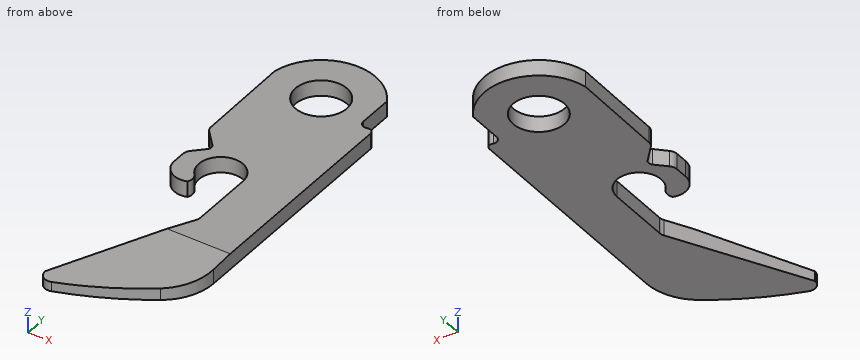
```python
from build123d import *

# Parameters (mm, degrees)
BOSS_EXTRUDE1_DEPTH = 1.27
SKETCH2_R           = 2.0701
CUT_EXTRUDE1_DEPTH  = 2.27
FILLET1_R           = 0.762
CUT_EXTRUDE2_DEPTH  = 10.452014607


with BuildPart() as part:
    # Sketch1 → Boss-Extrude1 (new body)
    with BuildSketch(Plane.XY):
        with BuildLine():
            Line((70.232354199, 59.177106463), (70.232354199, 40.597101988))
            ThreePointArc((70.232354199, 40.597101988), (69.734336591, 38.583930727), (68.355161738, 37.035138686))
            ThreePointArc((68.355161738, 37.035138686), (65.183135809, 35.174825007), (61.781607592, 33.777641675))
            ThreePointArc((61.781607592, 33.777641675), (61.096065134, 33.883458799), (60.780339592, 34.501101988))
            Line((60.780339592, 34.501101988), (66.266739592, 44.661101988))
            Line((66.266739592, 44.661101988), (66.266739592, 44.697700386))
            Line((66.266739592, 44.697700386), (66.266739592, 49.893501988))
            ThreePointArc((66.266739592, 49.893501988), (63.861714839, 51.557269988), (63.152989358, 48.720021988))
            ThreePointArc((63.152989358, 48.720021988), (63.340826318, 48.267953364), (63.214864671, 47.794896889))
            ThreePointArc((63.214864671, 47.794896889), (61.829181489, 47.989948212), (61.186739592, 49.233101988))
            Line((61.186739592, 49.233101988), (61.186739592, 50.249101988))
            ThreePointArc((61.186739592, 50.249101988), (61.245267671, 50.541969288), (61.411860998, 50.789847191))
            Line((61.411860998, 50.789847191), (62.237339742, 51.609423334))
            ThreePointArc((62.237339742, 51.609423334), (62.358185527, 51.888348141), (62.253539592, 52.173746074))
            Line((62.253539592, 52.173746074), (61.016973645, 53.551101988))
            Line((61.016973645, 53.551101988), (60.932739592, 61.477883946))
            ThreePointArc((60.932739592, 61.477883946), (64.518060362, 64.995788774), (69.060739592, 62.852369819))
            Line((69.060739592, 62.852369819), (69.060739592, 60.053501988))
            ThreePointArc((69.060739592, 60.053501988), (69.244620338, 59.662336155), (69.663143958, 59.554350892))
            ThreePointArc((69.663143958, 59.554350892), (70.049026383, 59.518542276), (70.232354199, 59.177106463))
        make_face()
    extrude(amount=BOSS_EXTRUDE1_DEPTH)

    # Sketch2 → Cut-Extrude1 (cut, through all)
    with BuildSketch(Plane.XY.offset(1.27)):
        with Locations((65.250739592, 60.663101988)):
            Circle(SKETCH2_R)
    extrude(amount=-CUT_EXTRUDE1_DEPTH, mode=Mode.SUBTRACT)

    # Fillet1
    fillet1_edges = [part.edges().sort_by_distance(p)[0] for p in [
        (66.266739592, 44.661101988, 0.635),
        (61.016973645, 53.551101988, 0.635),
    ]]
    fillet(fillet1_edges, radius=FILLET1_R)

    # Sketch3 → Cut-Extrude2 (cut, through all)
    with BuildSketch(Plane(origin=(70.232354199, 0, 0), x_dir=(0, 0, -1), z_dir=(1, 0, 0))):
        Polygon((-1.27, 33.739101988), (-0.762, 33.739101988), (-1.27, 42.563935936), align=None)
    extrude(amount=-CUT_EXTRUDE2_DEPTH, mode=Mode.SUBTRACT)


solid = part.part
```
Check sheet for the modelled part. Datum: model origin and axes. Units: mm. Give positions to 0.01 mm unless a question says otherwise; leave off trailing zeros. Order: outer loops, then holes, each group sorted by start corner. A loop starts at its lowest first (then second) coordinate and runs counter-clockwise, first axis right, second up. Notation, with made-up numbers: (67.25, 27.5) -> (85.25, 27.5) arc R22 cw to (85.25, 54.5) -> close; hole circle Ø10 at (23, 71.5). An arc over 180 degrees is marked (long way). Return JSON: item names as keys, results as strings.
1. Material ranges on probe 1 along Y at (x, z) = (61.75, 0.35); probe 2 along Y at (x, z) = (64, 0.7); probe 3 along X at (y, z) = (50.5, 0.25), recorded low to high. Write a range as [from, to].
From the geometry:
{"probe 1": "[33.77, 36.3], [48.05, 51.13], [52.73, 63.32]", "probe 2": "[34.62, 40.46], [51.6, 59.01], [62.31, 64.88]", "probe 3": "[61.23, 62.82], [66.16, 70.23]"}
2. Cross-section at D-D, the plane x = 68. Record the cut outline in (y, z).
From the geometry:
{"outline": "(36.8, 0) -> (64.09, 0) -> (64.09, 1.27) -> (42.56, 1.27) -> (36.8, 0.94) -> close"}
3. Cross-section at C-C, the plane y = 53. Record the cut outline in (x, z), plus the area to 3 significant figures.
From the geometry:
{"outline": "(61.51, 0) -> (70.23, 0) -> (70.23, 1.27) -> (61.51, 1.27) -> close", "area": "11.1 mm^2"}
4. Cross-section at B-B, the plane z = 0.4. Record the cut outline in (x, y), plus the area to 3 significant figures.
From the geometry:
{"outline": "(60.78, 34.5) arc R0.76 ccw to (61.78, 33.78) arc R26.16 ccw to (68.36, 37.04) arc R4.32 ccw to (70.23, 40.6) -> (70.23, 59.18) arc R0.41 ccw to (69.66, 59.55) arc R0.51 cw to (69.06, 60.05) -> (69.06, 62.85) arc R4.39 ccw to (60.93, 61.48) -> (61.01, 53.84) arc R0.76 ccw to (61.21, 53.34) -> (62.25, 52.17) arc R0.41 cw to (62.24, 51.61) -> (61.41, 50.79) arc R0.76 ccw to (61.19, 50.25) -> (61.19, 49.23) arc R1.52 ccw to (63.21, 47.79) arc R0.76 ccw to (63.15, 48.72) arc R1.78 cw (long way) to (66.27, 49.89) -> (66.27, 44.85) arc R0.76 cw to (66.18, 44.49) -> close; hole circle Ø4.14 at (65.25, 60.66)", "area": "188 mm^2"}
5. Cross-section at A-A, the plane x = 64.5. Record the cut outline in (y, z).
From the geometry:
{"outline": "(34.85, 0) -> (41.39, 0) -> (41.39, 1.2) -> (34.85, 0.83) -> close; (51.67, 0) -> (58.73, 0) -> (58.73, 1.27) -> (51.67, 1.27) -> close; (62.59, 0) -> (64.99, 0) -> (64.99, 1.27) -> (62.59, 1.27) -> close"}
6. Go/stop test with a flat-tipped pin: P1, Ø0.6, axis at y = 61, z = 0.5, coming from the +X side. Record where the tip stops, or that it passes through.
From the geometry:
{"P1": "x = 69.06"}
